from build123d import *

# Parameters (mm, degrees)
ESQUISSE1_W             = 34
ESQUISSE1_H             = 100.65
BOSS_EXTRU_1_DEPTH      = 12.5
ESQUISSE2_W             = 31
ESQUISSE2_H             = 97.65
ENL_V_MAT_EXTRU_1_DEPTH = 11
ESQUISSE5_R             = 2
BOSS_EXTRU_4_DEPTH      = 3
ESQUISSE6_R             = 1.2
BOSS_EXTRU_5_DEPTH      = 5.5
CONG_2_R                = 2
CONG_3_R                = 2
CONG_4_R                = 2
ESQUISSE7_W             = 7.5
ESQUISSE7_H             = 80
BOSS_EXTRU_6_DEPTH      = 1
ESQUISSE9_W             = 9.45
ESQUISSE9_H             = 80
BOSS_EXTRU_7_DEPTH      = 1.7
ESQUISSE10_W            = 4.6
ESQUISSE10_H            = 8.2
ESQUISSE10_W_2          = 4.5
ESQUISSE10_H_2          = 14
ENL_V_MAT_EXTRU_2_DEPTH = 3
ESQUISSE11_W            = 15.5
ESQUISSE11_H            = 4.6
ENL_V_MAT_EXTRU_3_DEPTH = 3
CONG_7_R                = 1


with BuildPart() as part:
    # Esquisse1 → Boss.-Extru.1 (new body)
    with BuildSketch(Plane.XY):
        with Locations((17, 50.325)):
            Rectangle(ESQUISSE1_W, ESQUISSE1_H)
    extrude(amount=BOSS_EXTRU_1_DEPTH)

    # Esquisse2 → Enlèv. mat.-Extru.1 (cut)
    with BuildSketch(Plane.XY.offset(12.5)):
        with Locations((17, 50.325)):
            Rectangle(ESQUISSE2_W, ESQUISSE2_H)
    extrude(amount=-ENL_V_MAT_EXTRU_1_DEPTH, mode=Mode.SUBTRACT)

    # Esquisse5 → Boss.-Extru.4 (add)
    with BuildSketch(Plane.XY.offset(1.5)):
        with Locations((5.5, 63.5)):
            Circle(ESQUISSE5_R)
        with Locations((28.5, 63.5)):
            Circle(ESQUISSE5_R)
        with Locations((5.5, 5.5)):
            Circle(ESQUISSE5_R)
        with Locations((28.5, 5.5)):
            Circle(ESQUISSE5_R)
    extrude(amount=BOSS_EXTRU_4_DEPTH)

    # Esquisse6 → Boss.-Extru.5 (add)
    with BuildSketch(Plane.XY.offset(1.5)):
        with Locations((5.5, 63.5)):
            Circle(ESQUISSE6_R)
        with Locations((28.5, 63.5)):
            Circle(ESQUISSE6_R)
        with Locations((5.5, 5.5)):
            Circle(ESQUISSE6_R)
        with Locations((28.5, 5.5)):
            Circle(ESQUISSE6_R)
    extrude(amount=BOSS_EXTRU_5_DEPTH)

    # Congé2
    cong_2_edges = [part.edges().sort_by_distance(p)[0] for p in [
        (34, 0, 6.25),
    ]]
    fillet(cong_2_edges, radius=CONG_2_R)

    # Congé3
    cong_3_edges = [part.edges().sort_by_distance(p)[0] for p in [
        (34, 100.65, 6.25),
    ]]
    fillet(cong_3_edges, radius=CONG_3_R)

    # Congé4
    cong_4_edges = [part.edges().sort_by_distance(p)[0] for p in [
        (16, 0, 0),
        (34, 50.325, 0),
        (33.414213562, 0.585786438, 0),
        (16, 100.65, 0),
        (33.414213562, 100.064213562, 0),
    ]]
    fillet(cong_4_edges, radius=CONG_4_R)

    # Esquisse7 → Boss.-Extru.6 (add)
    with BuildSketch(Plane.ZY):
        with Locations((7, 55.45)):
            Rectangle(ESQUISSE7_W, ESQUISSE7_H)
    extrude(amount=BOSS_EXTRU_6_DEPTH)

    # Esquisse9 → Boss.-Extru.7 (add)
    with BuildSketch(Plane.ZY.offset(1)):
        with Locations((6.725, 55.45)):
            Rectangle(ESQUISSE9_W, ESQUISSE9_H)
    extrude(amount=BOSS_EXTRU_7_DEPTH)

    # Esquisse10 → Enlèv. mat.-Extru.2 (cut)
    with BuildSketch(Plane.ZY.offset(-32.5)):
        with Locations((7.8, 55.9)):
            Rectangle(ESQUISSE10_W, ESQUISSE10_H)
        with Locations((7.8, 43.3)):
            Rectangle(ESQUISSE10_W, ESQUISSE10_H)
        with Locations((7.75, 14.3)):
            Rectangle(ESQUISSE10_W_2, ESQUISSE10_H_2)
    extrude(amount=-ENL_V_MAT_EXTRU_2_DEPTH, mode=Mode.SUBTRACT)

    # Esquisse11 → Enlèv. mat.-Extru.3 (cut)
    with BuildSketch(Plane(origin=(0, 1.5, 0), x_dir=(1, 0, 0), z_dir=(0, 1, 0))):
        with Locations((14.724178104, -7.8)):
            Rectangle(ESQUISSE11_W, ESQUISSE11_H)
    extrude(amount=-ENL_V_MAT_EXTRU_3_DEPTH, mode=Mode.SUBTRACT)

    # Congé7
    cong_7_edges = [part.edges().sort_by_distance(p)[0] for p in [
        (-2.7, 55.45, 2),
        (-2.7, 15.45, 6.725),
        (-2.7, 55.45, 11.45),
        (-2.7, 95.45, 6.725),
    ]]
    fillet(cong_7_edges, radius=CONG_7_R)


solid = part.part
Design review of the part built by this model. Coordinates are the model's own, in mm. A direction names the side the tool comes from. Coordinates: 2 decimals unless noted, no trailing zeros. Loops run counter-clockwise (first coordinate to the right, second up) from the corner with the lowest first, then second, coordinate; pieces in that order, holes last.
Item 1: Add section C-C (y = 45). Write out the cut boundary in (x, z).
Completed:
outline: (-2.7, 3) arc R1 ccw to (-1.7, 2) - (-1, 2) - (-1, 3.25) - (0, 3.25) - (0, 0) - (32, 0) arc R2 ccw to (34, 2) - (34, 5.5) - (32.5, 5.5) - (32.5, 1.5) - (1.5, 1.5) - (1.5, 12.5) - (0, 12.5) - (0, 10.75) - (-1, 10.75) - (-1, 11.45) - (-1.7, 11.45) arc R1 ccw to (-2.7, 10.45) - close; (32.5, 10.1) - (34, 10.1) - (34, 12.5) - (32.5, 12.5) - close
Item 2: Clearance check with flat-ended pins moving along their axes: pin 1 (1.9 mm diameter, centred on x = -1, z = 8, fed in from -Y); pin 2 (1.6 mm diameter, centred on y = 0.5, z = 8, fed in from -X); pin 3 (0.7 mm diameter, centred on x = 5.5, y = 5, fed in from +Z). State where each tip first meets the part, or that it passes through.
Completed:
pin 1: stops at y = 15.45
pin 2: stops at x = 0
pin 3: stops at z = 7
Item 3: Add section B-B (z = 9). Give the number of separate pieces and of enclosed holes in the cut face, and give its area (3 significant figures).
Completed:
separate pieces: 4
enclosed holes: 0
area: 540 mm2
Item 4: For faces 5 (the flat face through (-2.7, 56, 7)), 6 (the cylindrical face through (5.34, 64.69, 5.73)), list the 3-axis set-ups (+Z, -Z, +X, -X, +Y, -Y) from which the entire face can be reached by the end or side of a thin tool; tool diameter is ignored.
Completed:
face 5: +Z, -Z, -X, +Y, -Y
face 6: +Z
Item 5: Wall thickness on L1, parallel to Y at x = 25.5, z = 2.25; L2, parallel to X at y = 93, z = 8; L3, parallel to Y at x = 5, z = 4.25: over which ranges is each line inside the solid? List them lowest first.
Completed:
L1: y = 0 to 1.5, 99.15 to 100.65
L2: x = -2.7 to 1.5, 32.5 to 34
L3: y = 0 to 1.5, 3.56 to 7.44, 61.56 to 65.44, 99.15 to 100.65
Item 6: Add section D-D (y = 89.5). Write out the cut boundary in (x, z), and give its area (3 significant figures).
Completed:
outline: (-2.7, 3) arc R1 ccw to (-1.7, 2) - (-1, 2) - (-1, 3.25) - (0, 3.25) - (0, 0) - (32, 0) arc R2 ccw to (34, 2) - (34, 12.5) - (32.5, 12.5) - (32.5, 1.5) - (1.5, 1.5) - (1.5, 12.5) - (0, 12.5) - (0, 10.75) - (-1, 10.75) - (-1, 11.45) - (-1.7, 11.45) arc R1 ccw to (-2.7, 10.45) - close
area: 106 mm2
Item 7: Add section A-A (x = 19). Write out the cut boundary in (y, z), and give its area (3 significant figures).
Completed:
outline: (0, 2) arc R2 ccw to (2, 0) - (98.65, 0) arc R2 ccw to (100.65, 2) - (100.65, 12.5) - (99.15, 12.5) - (99.15, 1.5) - (1.5, 1.5) - (1.5, 5.5) - (0, 5.5) - close; (0, 10.1) - (1.5, 10.1) - (1.5, 12.5) - (0, 12.5) - close
area: 175 mm2
Item 8: Draft analysis for pull direction X (two halves, no side actions). For faces 1 (the cylindrical face through (28.34, 64.69, 5.73)), 2 (the cylindrical face through (33.43, 51, 0.6)), 3 (the flat face through (33, 51, 12.5)), 4 (the flat face through (5, 62, 4.5)), state which applies: pulls with the +X half, pulls with the -X half, needs draft (parallel to the pull), parting line crosses it, or undercut.
Completed:
face 1: undercut
face 2: pulls with the +X half
face 3: needs draft
face 4: undercut
